```python
from build123d import *

# Parameters (mm, degrees)
F0_W     = 215.9
F0_H     = 15.24
F1_DEPTH = 12.7
F2_R     = 7.7724
F3_DEPTH = 15.24
F4_R     = 3.175
F5_DEPTH = 15.241


with BuildPart() as f1:
    # F0 (on Front) → F1 (new body)
    with BuildSketch(Plane.XZ):
        Rectangle(F0_W, F0_H)
    extrude(amount=F1_DEPTH)

    # F2 (on face) → F3 (cut)
    with BuildSketch(Plane.XY.offset(7.62)):
        with Locations((-85.725, -8.89)):
            Circle(F2_R)
        with Locations((-66.675, -8.89)):
            Circle(F2_R)
        with Locations((-47.625, -8.89)):
            Circle(F2_R)
        with Locations((-28.575, -8.89)):
            Circle(F2_R)
        with Locations((-9.525, -8.89)):
            Circle(F2_R)
        with Locations((9.525, -8.89)):
            Circle(F2_R)
        with Locations((28.575, -8.89)):
            Circle(F2_R)
        with Locations((47.625, -8.89)):
            Circle(F2_R)
        with Locations((66.675, -8.89)):
            Circle(F2_R)
        with Locations((85.725, -8.89)):
            Circle(F2_R)
    extrude(amount=-F3_DEPTH, mode=Mode.SUBTRACT)

    # F4 (on face) → F5 (cut, through all)
    with BuildSketch(Plane.XY.offset(7.62)):
        with Locations((-100.603828, -6.168369)):
            Circle(F4_R)
        with Locations((100.603828, -6.168369)):
            Circle(F4_R)
    extrude(amount=-F5_DEPTH, mode=Mode.SUBTRACT)


solid = f1.part
```
The listing builds one solid part. Answer for the finished solid, in the listing's coordinates (mm). Give positions to 0.01 mm unless a question says otherwise; leave off trailing zeros. Order: outer loops, then holes, each group sorted by start corner. A loop starts at its lowest first (then second) coordinate and runs counter-clockwise, first axis right, second up.
1) Find section C-C on x = 69.5. Write down the section's boundary in (y, z).
Reported:
outline: (-1.65, -7.62) - (0, -7.62) - (0, 7.62) - (-1.65, 7.62) - close
2) Find section B-B on x = -11. Write down the section's boundary in (y, z).
Reported:
outline: (-1.26, -7.62) - (0, -7.62) - (0, 7.62) - (-1.26, 7.62) - close
3) Determine the mould class of faces 1 (the face through (-47.4, -1.12, 0.11)), 2 (the face through (19, -12.7, 0)), 3 (the face through (85.95, -1.12, 0.11)), 4 (the face through (-2, -5, -7.62)) for opening direction Y: pulls with the +Y half, pulls with the -Y half, needs draft (parallel to the pull), parting line crosses it, or undercut.
Reported:
face 1: undercut
face 2: pulls with the -Y half
face 3: undercut
face 4: needs draft
4) Given P1, Ø3, axis at x = -16, z = 4, coming from the -Y side; P2, Ø4, axis at x = -100.6, y = -6.17, coming from the +Z side; P3, Ø2, axis at x = -26, z = -4.5, coming from the -Y side, each flat-ended and moving along its own axis, determine where each tip first touches the part or whether it passes through.
Reported:
P1: stops at y = -12.7
P2: passes through
P3: stops at y = -1.99
5) Consider line 1 along Y through (x, z) = (81, -4.5); line 2 along Y through (x, z) = (12, -5.5). Determine where each line is inside the solid, lowest interval first.
Reported:
line 1: y = -2.72 to 0
line 2: y = -1.52 to 0
6) Find section A-A on z = -5.75. Write down the section's boundary in (x, y) (3 decimals), then the cut area to 3 significant figures.
Reported:
outline: (-107.95, -12.7) - (-92.5, -12.7) arc R7.772 cw (long way) to (-78.95, -12.7) - (-73.45, -12.7) arc R7.772 cw (long way) to (-59.9, -12.7) - (-54.4, -12.7) arc R7.772 cw (long way) to (-40.85, -12.7) - (-35.35, -12.7) arc R7.772 cw (long way) to (-21.8, -12.7) - (-16.3, -12.7) arc R7.772 cw (long way) to (-2.75, -12.7) - (2.75, -12.7) arc R7.772 cw (long way) to (16.3, -12.7) - (21.8, -12.7) arc R7.772 cw (long way) to (35.35, -12.7) - (40.85, -12.7) arc R7.772 cw (long way) to (54.4, -12.7) - (59.9, -12.7) arc R7.772 cw (long way) to (73.45, -12.7) - (78.95, -12.7) arc R7.772 cw (long way) to (92.5, -12.7) - (107.95, -12.7) - (107.95, 0) - (-107.95, 0) - close; hole circle Ø6.35 at (-100.604, -6.168); hole circle Ø6.35 at (100.604, -6.168)
area: 1,160 mm2
